The model under review builds one solid part; all positions refer to its coordinate system, in mm. A direction names the side the tool comes from. Coordinates: 2 decimals unless noted, no trailing zeros. Order: outer loops, then holes, each group sorted by start corner. A loop starts at its lowest first (then second) coordinate and runs counter-clockwise, first axis right, second up. Notation, with made-up numbers: M -16.75,69.5 L -2.75,69.5 A24 ccw -2.75,79.5 Z; hole C 68.5,24 d10. An arc over 180 degrees is marked long. One line per item, written item: value.
```python
from build123d import *

# Parameters (mm, degrees)
F0_W     = 14
F0_H     = 14
F0_W_2   = 15
F0_H_2   = 15
F1_DEPTH = 10


with BuildPart() as f1:
    # F0 (on Top) → F1 (new body)
    with BuildSketch(Plane.XY):
        Polygon((-21, -1.789773), (0, -1.789773), (0, 13.210227), (0, 19.210227), (-7, 19.210227), (-21, 19.210227), align=None)
        with Locations((-14, 26.210227)):
            Rectangle(F0_W, F0_H)
        with Locations((7.5, 5.710227)):
            Rectangle(F0_W_2, F0_H_2)
    extrude(amount=F1_DEPTH)


solid = f1.part
```
(1) We need section C-C, the plane x = -4. State the section outline as (y, z) points, plus the area to 3 significant figures.
Geometry results:
outline: M -1.79,0 L 19.21,0 L 19.21,10 L -1.79,10 Z
area: 210 mm2
(2) Tool access review of faces 1 (the flat face through (-7, 12, 0)), 2 (the flat face through (0, 16, 5)): name each direction out of +Z, -Z, +X, -X, +Y, -Y from which nothing blocks a thin tool from reaching the whole face with its end or side.
Geometry results:
face 1: -Z, +X, -X, +Y, -Y
face 2: +Z, -Z, +X, +Y
(3) We need section A-A, the plane z = 4.5. State the section outline as (x, y) points.
Geometry results:
outline: M -21,-1.79 L 15,-1.79 L 15,13.21 L 0,13.21 L 0,19.21 L -7,19.21 L -7,33.21 L -21,33.21 Z
(4) Insertion check: pin 1 Ø5 at (y, z) = (26, 7) entering from +X; pin 2 Ø3.5 at (x, z) = (-2.5, 5.5) entering from +Y; pin 3 Ø5 at (y, z) = (19, 4.5) entering from +X. Each pin has a flat end and moves straight along its axis. Give the tip position at first contact, or say it passes through.
Geometry results:
pin 1: stops at x = -7
pin 2: stops at y = 19.21
pin 3: stops at x = 0
(5) We need section B-B, the plane y = 17.5. State the section outline as (x, z) points.
Geometry results:
outline: M -21,0 L 0,0 L 0,10 L -21,10 Z
(6) For L1, parallel to Y at x = -3, z = 7; L2, parallel to X at y = 29, z = 0.75; L3, parallel to Y at x = 9, z = 9.25, list the stretches that pass through material, from the lowest coordinate up.
Geometry results:
L1: y = -1.79 to 19.21
L2: x = -21 to -7
L3: y = -1.79 to 13.21
